Design review of the part built by this model. Coordinates are the model's own, in mm. Face numbers are marked on the shaded views. Give positions to 0.01 mm unless a question says otherwise; leave off trailing zeros. Write each loop counter-clockwise with the first axis right and the second up, starting at its lowest first coordinate (ties: lowest second). Pieces come first, ordered by that corner, then holes.
```python
from build123d import *

# Parameters (mm, degrees)
SKETCH1_W                             = 50
SKETCH1_H                             = 30
BOSS_EXTRUDE1_DEPTH                   = 13
TAP_DRILL_FOR_5_16_18_HELICOIL1_D     = 8.4328
TAP_DRILL_FOR_5_16_18_HELICOIL1_DEPTH = 129.53
TAP_DRILL_FOR_5_16_18_HELICOIL1_TIP   = 2.533468714
F_10_CLEARANCE_HOLE1_D                = 4.9784
F_10_CLEARANCE_HOLE1_DEPTH            = 129.53
F_10_CLEARANCE_HOLE1_TIP              = 1.495662253


with BuildPart() as part:
    # Sketch1 → Boss-Extrude1 (new body)
    with BuildSketch(Plane.XY):
        Rectangle(SKETCH1_W, SKETCH1_H)
    extrude(amount=BOSS_EXTRUDE1_DEPTH)

    # Tap Drill for 5/16-18 Helicoil1
    with Locations(Plane(origin=(0, 0, 0), x_dir=(-1, 0, 0), z_dir=(0, 0, -1))):
        with Locations((0, 0)):
            Hole(TAP_DRILL_FOR_5_16_18_HELICOIL1_D / 2, depth=TAP_DRILL_FOR_5_16_18_HELICOIL1_DEPTH)
            with Locations((0, 0, -(TAP_DRILL_FOR_5_16_18_HELICOIL1_DEPTH + TAP_DRILL_FOR_5_16_18_HELICOIL1_TIP / 2))):  # 118° drill point
                Cone(0, TAP_DRILL_FOR_5_16_18_HELICOIL1_D / 2, TAP_DRILL_FOR_5_16_18_HELICOIL1_TIP, mode=Mode.SUBTRACT)

    # #10 Clearance Hole1
    with Locations(Plane(origin=(0, 0, 0), x_dir=(-1, 0, 0), z_dir=(0, 0, -1))):
        with Locations((-16, 0), (16, 0)):
            Hole(F_10_CLEARANCE_HOLE1_D / 2, depth=F_10_CLEARANCE_HOLE1_DEPTH)
            with Locations((0, 0, -(F_10_CLEARANCE_HOLE1_DEPTH + F_10_CLEARANCE_HOLE1_TIP / 2))):  # 118° drill point
                Cone(0, F_10_CLEARANCE_HOLE1_D / 2, F_10_CLEARANCE_HOLE1_TIP, mode=Mode.SUBTRACT)


solid = part.part
```
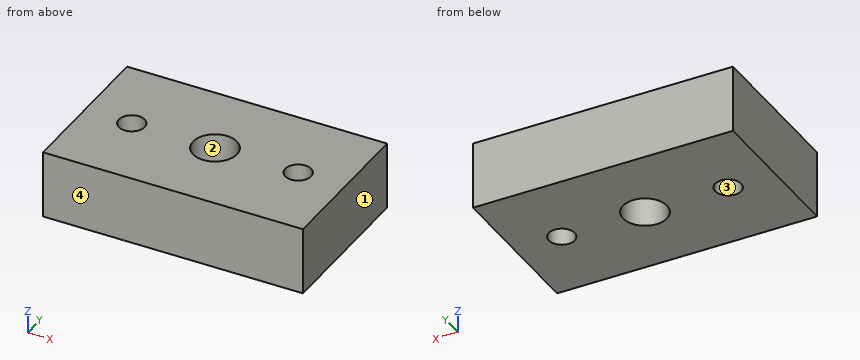
(1) Consider section D-D, the plane x = 0. Give the boundary of the cut face in (y, z).
Resolved:
outline: (-15, 0) - (-4.22, 0) - (-4.22, 13) - (-15, 13) - close; (4.22, 0) - (15, 0) - (15, 13) - (4.22, 13) - close
(2) Consider section B-B, the plane y = 0. Give the boundary of the cut face in (x, z).
Resolved:
outline: (-25, 0) - (-18.49, 0) - (-18.49, 13) - (-25, 13) - close; (-13.51, 0) - (-4.22, 0) - (-4.22, 13) - (-13.51, 13) - close; (4.22, 0) - (13.51, 0) - (13.51, 13) - (4.22, 13) - close; (18.49, 0) - (25, 0) - (25, 13) - (18.49, 13) - close
(3) Mouldability with a two-part tool opening along Y and no side actions: class the marked faces 1, 2, 3 and 4 as pulls with the +Y half, pulls with the -Y half, needs draft (parallel to the pull), parting line crosses it, or undercut.
Resolved:
face 1: needs draft
face 2: undercut
face 3: undercut
face 4: pulls with the -Y half
(4) To check wall thickness, follow L1, parallel to Y at x = 16, z = 4.5; L2, parallel to Y at x = 0, z = 9.5; L3, parallel to X at y = 1, z = 2.75. State the ranges of each line that lie inside material, in increasing order.
Resolved:
L1: y = -15 to -2.49, 2.49 to 15
L2: y = -15 to -4.22, 4.22 to 15
L3: x = -25 to -18.28, -13.72 to -4.1, 4.1 to 13.72, 18.28 to 25
(5) Consider section C-C, the plane z = 9.25. Give the boundary of the cut face in (x, y), then the cut area to 3 significant figures.
Resolved:
outline: (-25, -15) - (25, -15) - (25, 15) - (-25, 15) - close; hole circle Ø4.98 at (-16, 0); hole circle Ø8.43 at (0, 0); hole circle Ø4.98 at (16, 0)
area: 1,410 mm2
(6) Consider section A-A, the plane x = 16. Give the boundary of the cut face in (y, z), then the cut area to 3 significant figures.
Resolved:
outline: (-15, 0) - (-2.49, 0) - (-2.49, 13) - (-15, 13) - close; (2.49, 0) - (15, 0) - (15, 13) - (2.49, 13) - close
area: 325 mm2
